Can you work these out from the model? Positions are in its coordinate system, mm. A direction names the side the tool comes from. Round coordinates to 2 decimals unless told otherwise and drop trailing zeros. Write each loop counter-clockwise with the first axis right and the second up, starting at its lowest first coordinate (ties: lowest second). Pieces come first, ordered by that corner, then holes.
Q1. If we section it at D-D (z = 12): Please give me the cut outline in (x, y), plus the area to 3 significant figures.
Q2. Please list where these lines run through material, in increasing order: line 1 along X through (y, z) = (-21, 18); line 2 along Z through (x, y) = (-9, 0.5); line 3 along Z through (x, y) = (13.1, -22).
Q3. If we section it at A-A (z = 4.5): Please give me the cut outline in (x, y), plus the area to 3 significant figures.
Q4. For faces 5 (the flat face through (-3, 5, 2)), 6 (the flat face through (10, -17.6, 14.8)), 7 (the flat face through (-12.5, 0, 23)), 8 (the flat face through (15, -16, 12)), 9 (the flat face through (12.5, 0, 1)), which set-ups out of +Z, -Z, +X, -X, +Y, -Y let a thin tool reach every point of the face, with its end or its side?
Q5. If we section it at C-C (y = 0): Please give me the cut outline in (x, z), plus the area to 3 significant figures.
Q6. We'd pull the mould along Z, two halves only. Please class faces 1 (the cylindrical face through (12, -18, 15)), 2 (the flat face through (-12.5, 0, 1)), 3 (the flat face through (13, -10, 12)), 4 (the flat face through (-0.2, -5.3, 24)): +Z half, -Z half, draft (parallel to the pull), parting line (faces both ways), or undercut.
Q7. I'm going to push flat-ended pins straight in: pin 1 Ø8 at (y, z) = (5.5, 6.5) entering from -X; pin 2 Ø1 at (y, z) = (-1.5, 22.5) entering from -X; pin 3 Ø2 at (x, z) = (-1.5, 22.5) entering from -Y; pin 4 Ø4 at (x, z) = (-13.5, 13.5) entering from +Y. Where does each tip first touch, or does it pass through?
Q8. If we section it at B-B (x = 5.5): Please give me the cut outline in (y, z).
from build123d import *

# Parameters (mm, degrees)
SKETCH1_R           = 5
BOSS_EXTRUDE1_DEPTH = 2
BOSS_EXTRUDE2_DEPTH = 12
SKETCH2_R           = 5
CUT_EXTRUDE1_DEPTH  = 48


with BuildPart() as part:
    # Sketch1 → Boss-Extrude1 (new body)
    with BuildSketch(Plane.XY):
        Polygon((-10, -10), (10, -10), (12.5, -10), (12.5, 10), (-12.5, 10), (-12.5, -10), align=None)
        Circle(SKETCH1_R, mode=Mode.SUBTRACT)
    boss_extrude1 = extrude(amount=BOSS_EXTRUDE1_DEPTH)

    # Sketch1<3> → Boss-Extrude2 (add)
    with BuildSketch(Plane.XY):
        Polygon((10, -10), (10, -30), (15, -30), (15, -10), (12.5, -10), align=None)
        Polygon((-10, -30), (-10, -10), (-12.5, -10), (-15, -10), (-15, -30), align=None)
    boss_extrude2 = extrude(amount=BOSS_EXTRUDE2_DEPTH)

    # Mirror1: Boss-Extrude2 across plane
    add(boss_extrude2.mirror(Plane.XY.offset(12)))

    # Mirror2: Boss-Extrude1 across plane
    add(boss_extrude1.mirror(Plane.XY.offset(12)))

    # Sketch2 → Cut-Extrude1 (cut)
    with BuildSketch(Plane.ZY.offset(15)):
        with Locations(Location((12, -22, 0), (0, 0, 270))):
            Circle(SKETCH2_R)
    extrude(amount=-CUT_EXTRUDE1_DEPTH, mode=Mode.SUBTRACT)


solid = part.part
A:
1. outline: (-15, -30) - (-10, -30) - (-10, -27) - (-15, -27) - close; (-15, -17) - (-10, -17) - (-10, -10) - (-15, -10) - close; (10, -30) - (15, -30) - (15, -27) - (10, -27) - close; (10, -17) - (15, -17) - (15, -10) - (10, -10) - close
1. area: 100 mm2
2. line 1: x = -15 to -10, 10 to 15
2. line 2: z = 0 to 2, 22 to 24
2. line 3: z = 0 to 7, 17 to 24
3. outline: (-15, -30) - (-10, -30) - (-10, -10) - (-15, -10) - close; (10, -30) - (15, -30) - (15, -10) - (10, -10) - close
3. area: 200 mm2
4. face 5: +X, -X, +Y
4. face 6: +Z, -Z, -Y
4. face 7: +Z, -Z, -X, +Y
4. face 8: +Z, -Z, +X, +Y, -Y
4. face 9: +Z, -Z, +X, +Y
5. outline: (-12.5, 0) - (-5, 0) - (-5, 2) - (-12.5, 2) - close; (-12.5, 22) - (-5, 22) - (-5, 24) - (-12.5, 24) - close; (5, 0) - (12.5, 0) - (12.5, 2) - (5, 2) - close; (5, 22) - (12.5, 22) - (12.5, 24) - (5, 24) - close
5. area: 60.0 mm2
6. face 1: undercut
6. face 2: draft
6. face 3: undercut
6. face 4: +Z half
7. pin 1: passes through
7. pin 2: stops at x = -12.5
7. pin 3: stops at y = -10
7. pin 4: stops at y = -10
8. outline: (-10, 0) - (10, 0) - (10, 2) - (-10, 2) - close; (-10, 22) - (10, 22) - (10, 24) - (-10, 24) - close
